Build history of the part. All positions in model axes, mm. Face numbers are marked on the shaded views. Give positions to 0.01 mm unless a question says otherwise; leave off trailing zeros. Write each loop counter-clockwise with the first axis right and the second up, starting at its lowest first coordinate (ties: lowest second). Pieces come first, ordered by that corner, then holes. Notation, with made-up numbers: (1, 0.25) -> (50, 0.25) arc R21 cw to (50, 7.25) -> close; hole circle Ø10 at (49, -32). An arc over 180 degrees is marked (long way). Write item = value, one per line. Start each with the question number.
Q1. Saw through at A-A, the plane x = 43. List the corners of the cut face in (y, z).
Q2. Saw through at C-C, the plane y = 46.5. List the corners of the cut face in (x, z), then the cut area to 3 significant figures.
Q3. Drop flat-ended pins along their axis: P1, Ø2, axis at y = 27.5, z = 12, coming from the -X side; P2, Ø6, axis at y = 7.5, z = 23, coming from the +X side; P3, Ø4, axis at y = 37.5, z = 7, coming from the +X side. Give the stop position or say it passes through.
Q4. Saw through at B-B, the plane y = 18.5. List the corners of the cut face in (x, z).
Q5. Mould opens along Z. For the marked faces 1, 2, 3 and 4 say: pulls with the +Z half, pulls with the -Z half, needs draft (parallel to the pull), parting line crosses it, or undercut.
Q6. Wall check: line 1 (Y direction, x = 7, z = 4); line 2 (Z direction, x = 20, y = 6.5); line 3 (Z direction, x = 39, y = 38). Give the ranges that are in metal, low to high.
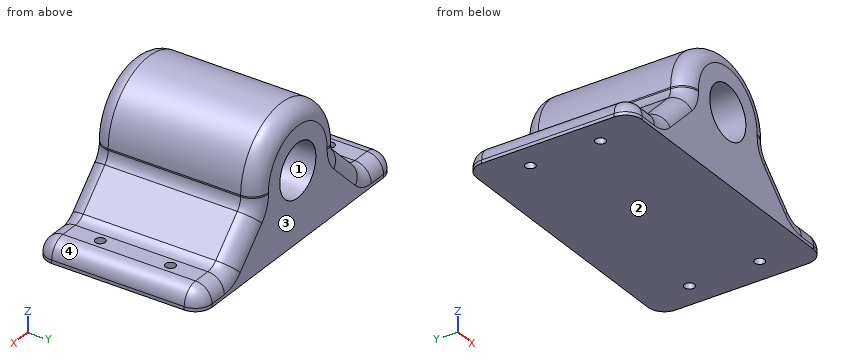
from build123d import *

# Parameters (mm, degrees)
SKETCH1_W           = 86
SKETCH1_H           = 50
BOSS_EXTRUDE2_DEPTH = 6
BOSS_EXTRUDE3_DEPTH = 50
SKETCH4_R           = 8
CUT_EXTRUDE1_DEPTH  = 121
BOSS_EXTRUDE5_DEPTH = 50
BOSS_EXTRUDE6_DEPTH = 50
FILLET1_R           = 5
FILLET2_R           = 5
FILLET3_R           = 5
FILLET4_R           = 5
FILLET5_R           = 5
SKETCH7_R           = 1.5
CUT_EXTRUDE2_DEPTH  = 50
SKETCH8_R           = 1.5
CUT_EXTRUDE4_DEPTH  = 50


with BuildPart() as part:
    # Sketch1 → Boss-Extrude2 (new body)
    with BuildSketch(Plane.XY):
        with Locations((43, 25)):
            Rectangle(SKETCH1_W, SKETCH1_H)
    extrude(amount=BOSS_EXTRUDE2_DEPTH)

    # Sketch2 → Boss-Extrude3 (add)
    with BuildSketch(Plane(origin=(0, 0, 0), x_dir=(-1, 0, 0), z_dir=(0, -1, 0))):
        with BuildLine():
            Line((-61, -21), (-61, -6))
            Line((-61, -6), (-25, -6))
            Line((-25, -6), (-25, -21))
            ThreePointArc((-25, -21), (-43, -39), (-61, -21))
        make_face()
    extrude(amount=-BOSS_EXTRUDE3_DEPTH)

    # Sketch4 → Cut-Extrude1 (cut)
    with BuildSketch(Plane(origin=(0, 0, 0), x_dir=(-1, 0, 0), z_dir=(0, -1, 0))):
        with Locations(Location((-43, -21, 0), (0, 0, 90))):
            Circle(SKETCH4_R)
    extrude(amount=-CUT_EXTRUDE1_DEPTH, mode=Mode.SUBTRACT)

    # Sketch5 → Boss-Extrude5 (add)
    with BuildSketch(Plane(origin=(0, 0, 0), x_dir=(-1, 0, 0), z_dir=(0, -1, 0))):
        Polygon((-61, -6), (-73.5, -6), (-61, -18.5), align=None)
    extrude(amount=-BOSS_EXTRUDE5_DEPTH)

    # Sketch6 → Boss-Extrude6 (add)
    with BuildSketch(Plane(origin=(0, 0, 0), x_dir=(-1, 0, 0), z_dir=(0, -1, 0))):
        Polygon((-25, -6), (-12.5, -6), (-25, -18.5), align=None)
    extrude(amount=-BOSS_EXTRUDE6_DEPTH)

    # Fillet1
    fillet1_edges = [part.edges().sort_by_distance(p)[0] for p in [
        (86, 25, 6),
    ]]
    fillet(fillet1_edges, radius=FILLET1_R)

    # Fillet2
    fillet2_edges = [part.edges().sort_by_distance(p)[0] for p in [
        (73.5, 25, 6),
    ]]
    fillet(fillet2_edges, radius=FILLET2_R)

    # Fillet3
    fillet3_edges = [part.edges().sort_by_distance(p)[0] for p in [
        (61, 25, 18.5),
    ]]
    fillet(fillet3_edges, radius=FILLET3_R)

    # Fillet4
    fillet4_edges = [part.edges().sort_by_distance(p)[0] for p in [
        (25, 25, 18.5),
        (0, 25, 6),
        (12.5, 25, 6),
    ]]
    fillet(fillet4_edges, radius=FILLET4_R)

    # Fillet5
    fillet5_edges = [part.edges().sort_by_distance(p)[0] for p in [
        (43, 0, 39),
        (61, 0, 20.785533906),
        (43, 50, 39),
        (61, 50, 20.785533906),
        (78.285533906, 50, 6),
        (86, 50, 0.5),
        (84.535533906, 50, 4.535533906),
        (86, 0, 0.5),
        (84.535533906, 0, 4.535533906),
        (78.285533906, 0, 6),
        (67.25, 0, 12.25),
        (67.25, 50, 12.25),
        (73.65765065, 0, 6.380602337),
        (73.65765065, 50, 6.380602337),
        (61.380602337, 0, 18.65765065),
        (61.380602337, 50, 18.65765065),
        (18.75, 0, 12.25),
        (18.75, 50, 12.25),
        (7.714466094, 50, 6),
        (7.714466094, 0, 6),
        (25, 50, 20.785533906),
        (25, 0, 20.785533906),
        (0, 0, 0.5),
        (1.464466094, 0, 4.535533906),
        (0, 50, 0.5),
        (1.464466094, 50, 4.535533906),
        (12.34234935, 0, 6.380602337),
        (12.34234935, 50, 6.380602337),
        (24.619397663, 0, 18.65765065),
        (24.619397663, 50, 18.65765065),
    ]]
    fillet(fillet5_edges, radius=FILLET5_R)

    # Sketch7 → Cut-Extrude2 (cut)
    with BuildSketch(Plane.XY.offset(6)):
        with Locations((7.714466094, 35.601677871)):
            Circle(SKETCH7_R)
        with Locations((7.714466094, 14.398322129)):
            Circle(SKETCH7_R)
    extrude(amount=-CUT_EXTRUDE2_DEPTH, mode=Mode.SUBTRACT)

    # Sketch8 → Cut-Extrude4 (cut)
    with BuildSketch(Plane.XY.offset(6)):
        with Locations((78.285533906, 35.60168)):
            Circle(SKETCH8_R)
        with Locations((78.285533906, 14.39832)):
            Circle(SKETCH8_R)
    extrude(amount=-CUT_EXTRUDE4_DEPTH, mode=Mode.SUBTRACT)


solid = part.part
Report:
q1.outline = (0, 0) -> (50, 0) -> (50, 13) -> (0, 13) -> close; (0, 29) -> (50, 29) -> (50, 34) arc R5 ccw to (45, 39) -> (5, 39) arc R5 ccw to (0, 34) -> close
q2.outline = (0.23, 0) -> (85.77, 0) -> (85.77, 1) arc R4.77 ccw to (81, 5.77) -> (75.57, 5.77) arc R5.23 cw to (71.87, 7.3) -> (62.3, 16.87) arc R5.23 cw to (60.77, 20.57) -> (60.77, 21) arc R17.77 ccw to (25.23, 21) -> (25.23, 20.57) arc R5.23 cw to (23.7, 16.87) -> (14.13, 7.3) arc R5.23 cw to (10.43, 5.77) -> (5, 5.77) arc R4.77 ccw to (0.23, 1) -> close; hole circle Ø16 at (43, 21)
q2.area = 1,480 mm2
q3.P1 = 17.5
q3.P2 = 61.03
q3.P3 = 84
q4.outline = (0, 0) -> (86, 0) -> (86, 1) arc R5 ccw to (81, 6) -> (75.57, 6) arc R5 cw to (72.04, 7.46) -> (62.46, 17.04) arc R5 cw to (61, 20.57) -> (61, 21) arc R18 ccw to (25, 21) -> (25, 20.57) arc R5 cw to (23.54, 17.04) -> (13.96, 7.46) arc R5 cw to (10.43, 6) -> (5, 6) arc R5 ccw to (0, 1) -> close; hole circle Ø16 at (43, 21)
q5.face_1 = undercut
q5.face_2 = pulls with the -Z half
q5.face_3 = needs draft
q5.face_4 = pulls with the +Z half
q6.line_1 = 1 to 13.08, 15.72 to 34.28, 36.92 to 49
q6.line_2 = 0 to 13.5
q6.line_3 = 0 to 14.07, 27.93 to 38.55
